Input: part model. Units: mm. Frame: model coordinates. Coordinates: 2 decimals unless noted, no trailing zeros. Order: outer loops, then holes, each group sorted by start corner. A loop starts at its lowest first (then second) coordinate and runs counter-clockwise, first axis right, second up. Notation, with made-up numbers: (-13.75, 81) - (0.25, 81) arc R35 cw to (0.25, 117) - close; hole circle Ø7 at (38.5, 3.25). An arc over 180 degrees is marked (long way). Answer as CSV lines item,"result". Start each with the question number.
Item 1: Section A-A (y = 10). Output: boundary loops of the cut face in (x, z), and give its area (3 significant figures).
Item 2: First-contact query: pin 1 (6 mm diameter, centred on x = 0, y = 10, fed in from -Z). Flat tip, straight axial feed; report the tip coordinate or a pass-through.
Item 3: Section B-B (z = 74). Output: boundary loops of the cut face in (x, y).
Item 4: Material intervals for line 1 along X through (y, z) = (9.75, 6); line 2 along Y through (x, z) = (0, -5.5); line 3 along X through (y, z) = (14.5, -167.5), sorted ascending.
Item 5: Section C-C (x = 150). Output: boundary loops of the cut face in (y, z).
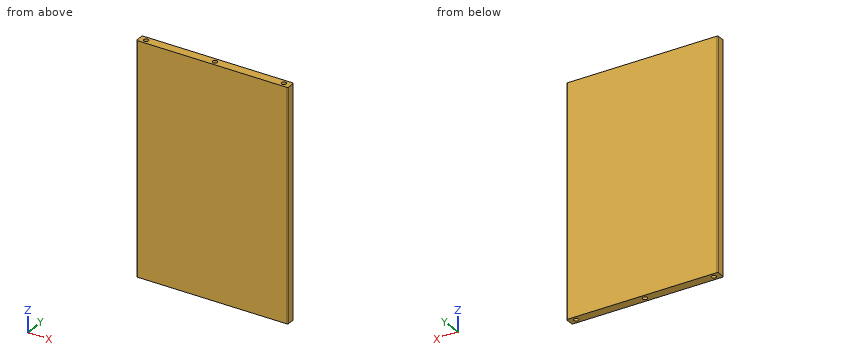
from build123d import *

# Parameters (mm, degrees)
SKETCH1_W           = 330
SKETCH1_H           = 500
BOSS_EXTRUDE1_DEPTH = 20
SKETCH2_R           = 5
CUT_EXTRUDE1_DEPTH  = 527.901319034
FILLET1_R           = 2


with BuildPart() as part:
    # Sketch1 → Boss-Extrude1 (new body)
    with BuildSketch(Plane(origin=(0, 0, 0), x_dir=(1, 0, 0), z_dir=(0, 1, 0))):
        Rectangle(SKETCH1_W, SKETCH1_H)
    extrude(amount=BOSS_EXTRUDE1_DEPTH)

    # Sketch2 → Cut-Extrude1 (cut, through all)
    with BuildSketch(Plane.XY.offset(250)):
        with Locations((0, 10)):
            Circle(SKETCH2_R)
        with Locations((-150, 10)):
            Circle(SKETCH2_R)
        with Locations((150, 10)):
            Circle(SKETCH2_R)
    extrude(amount=-CUT_EXTRUDE1_DEPTH, mode=Mode.SUBTRACT)

    # Fillet1
    fillet1_edges = [part.edges().sort_by_distance(p)[0] for p in [
        (-165, 20, 0),
        (165, 20, 0),
        (-165, 0, 0),
        (165, 0, 0),
    ]]
    fillet(fillet1_edges, radius=FILLET1_R)


solid = part.part
Determined:
1,outline,"(-165, -250) - (-155, -250) - (-155, 250) - (-165, 250) - close; (-145, -250) - (-5, -250) - (-5, 250) - (-145, 250) - close; (5, -250) - (145, -250) - (145, 250) - (5, 250) - close; (155, -250) - (165, -250) - (165, 250) - (155, 250) - close"
1,area,"150,000 mm^2"
2,pin 1,"passes through"
3,outline,"(-165, 2) arc R2 ccw to (-163, 0) - (163, 0) arc R2 ccw to (165, 2) - (165, 18) arc R2 ccw to (163, 20) - (-163, 20) arc R2 ccw to (-165, 18) - close; hole circle Ø10 at (-150, 10); hole circle Ø10 at (0, 10); hole circle Ø10 at (150, 10)"
4,line 1,"x = -165 to -154.99, -145.01 to -4.99, 4.99 to 145.01, 154.99 to 165"
4,line 2,"y = 0 to 5, 15 to 20"
4,line 3,"x = -165 to -152.18, -147.82 to -2.18, 2.18 to 147.82, 152.18 to 165"
5,outline,"(0, -250) - (5, -250) - (5, 250) - (0, 250) - close; (15, -250) - (20, -250) - (20, 250) - (15, 250) - close"
